Verification items for the finished model (mm, model axes). Face numbers are marked on the shaded views. Coordinates: 2 decimals unless noted, no trailing zeros. Order: outer loops, then holes, each group sorted by start corner. A loop starts at its lowest first (then second) coordinate and runs counter-clockwise, first axis right, second up. Notation, with made-up numbers: (79, -34.75) -> (129, -34.75) arc R31 cw to (129, -7.75) -> close; hole circle Ø9 at (75.25, -6). An arc over 180 degrees is marked (long way). Write item = value, one per line. Start each with the question number.
1. Go/stop test with flat-tipped pins: P1, Ø1.5, axis at x = -16.5, y = -5.5, coming from the -Z side; P2, Ø1.5, axis at x = 15.5, z = 0.5, coming from the +Y side; P3, Ø8, axis at x = -12, y = -16.5, coming from the +Z side; P4, Ø2, axis at y = -17, z = -1, coming from the +X side. Record where each tip stops, or that it passes through.
2. Cross-section at C-C on z = 0.6. Record the cut outline in (x, y), plus the area to 3 significant figures.
3. Thickness scan on line 1 along Y through (x, z) = (0, -0.3); line 2 along X through (y, z) = (-0.5, -0.8); line 3 along X through (y, z) = (-1.5, 1.9). Record the ranges inside material, lowest first. Write a range as from..to.
4. Release check for a two-part mould opening along Y. For the marked faces 1 and 2 record: +Y half, -Y half, draft (parallel to the pull), parting line (faces both ways), or undercut.
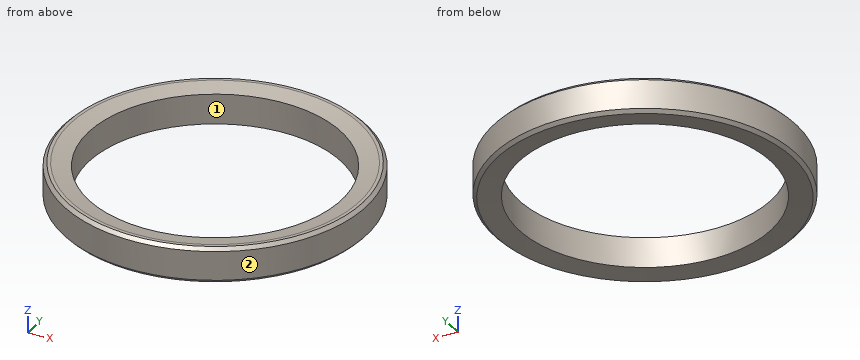
from build123d import *

# Parameters (mm, degrees)
CHAMFER1_SIZE = 0.5


with BuildPart() as part:
    # Sketch2 → Revolve1 (revolve)
    with BuildSketch(Plane(origin=(0, 0, 0), x_dir=(0, 0, -1), z_dir=(1, 0, 0)), mode=Mode.PRIVATE) as revolve1_sk:
        Polygon((-2.810478001, 22.7), (2.559521999, 22.7), (2.559521999, 22.2), (2.265464537, 18.95), (-2.265464537, 18.95), (-2.810478001, 21.7), align=None)
    revolve(revolve1_sk.sketch.rotate(Axis((0, 0, -1.408758661), (0, 0, 1)), 90), axis=Axis((0, 0, -1.408758661), (0, 0, 1)))

    # Chamfer1
    chamfer1_edges = [part.edges().sort_by_distance(p)[0] for p in [
        (22.7, 0, 2.810478001),
        (22.7, 0, -2.559521999),
    ]]
    chamfer(chamfer1_edges, length=CHAMFER1_SIZE - 0.0001)  # a hair under: the kernel refuses the full size


solid = part.part
Worked out:
q1.P1 = through
q1.P2 = 17.25
q1.P3 = 2.81
q1.P4 = 16.1
q2.outline = circle Ø45.4 at (0, 0); hole circle Ø37.9 at (0, 0)
q2.area = 491 mm²
q3.line_1 = -22.7..-18.95, 18.95..22.7
q3.line_2 = -22.69..-18.94, 18.94..22.69
q3.line_3 = -22.65..-18.89, 18.89..22.65
q4.face_1 = undercut
q4.face_2 = parting line
